Read the model definition and answer for the solid it produces. Units are mm, in the model's axes. Face numbers are marked on the shaded views. Coordinates: 2 decimals unless noted, no trailing zeros. Write each loop counter-clockwise with the first axis right and the second up, starting at its lowest first coordinate (ties: lowest second). Pieces come first, ordered by that corner, then holes.
1) The part is cut by section C-C (z = 1.5). Determine the outline of the cut face in (x, y).
2) Each of these flat-tipped pins is pushed along its axis until it touches: pin 1 Ø5 at (x, y) = (95.5, 15.5) entering from +Z; pin 2 Ø6 at (y, z) = (24.5, 3) entering from +X. Where does it stop, or does it pass through?
3) The part is cut by section A-A (x = 15). Determine the outline of the cut face in (y, z), then the cut area to 3 significant figures.
4) Determine the mould class of the marked faces 1, 2 and 3 for opening direction Z: +Z half, -Z half, draft (parallel to the pull), parting line (faces both ways), or undercut.
5) The part is cut by section D-D (y = 27). Determine the outline of the cut face in (x, z).
6) The part is cut by section B-B (y = 15). Determine the outline of the cut face in (x, z).
7) Find the intervals of material crossed by line 1 (Z direction, x = 46.5, y = 12); line 2 (Y direction, x = 15, z = 1); line 3 (Y direction, x = 9, z = 2.25), in increasing order.
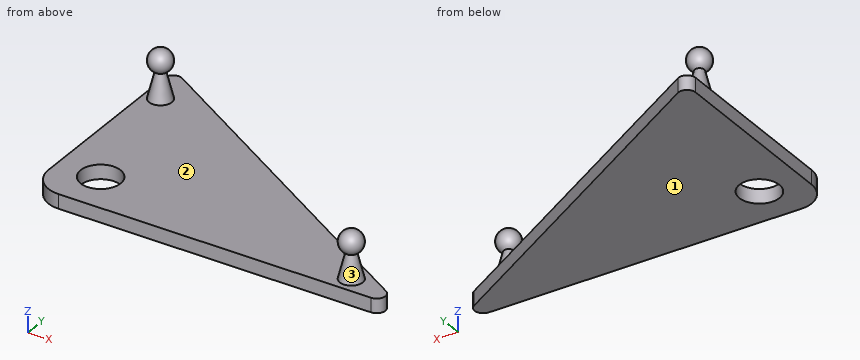
from build123d import *

# Parameters (mm, degrees)
ESTRUSIONE_ESTRUSIONE1_DEPTH = 5
SCHIZZO2_R                   = 7
TAGLIO_ESTRUSIONE1_DEPTH     = 152.6871781
RACCORDO1_R                  = 10
SCHIZZO3_R                   = 4
ESTRUSIONE_ESTRUSIONE2_DEPTH = 10
ESTRUSIONE_ESTRUSIONE2_TAPER = 14
RACCORDO2_R                  = 3
SCHIZZO6_R                   = 4
ESTRUSIONE_ESTRUSIONE3_DEPTH = 10
ESTRUSIONE_ESTRUSIONE3_TAPER = 14


with BuildPart() as part:
    # Schizzo1 → Estrusione-Estrusione1 (new body)
    with BuildSketch(Plane.XY):
        Polygon((0, 0), (0, 78), (130, 0), align=None)
    extrude(amount=ESTRUSIONE_ESTRUSIONE1_DEPTH)

    # Schizzo2 → Taglio-Estrusione1 (cut, through all)
    with BuildSketch(Plane(origin=(0, 0, 0), x_dir=(-1, 0, 0), z_dir=(0, 0, -1))):
        with Locations((-15, 15)):
            Circle(SCHIZZO2_R)
    extrude(amount=-TAGLIO_ESTRUSIONE1_DEPTH, mode=Mode.SUBTRACT)

    # Raccordo1
    raccordo1_edges = [part.edges().sort_by_distance(p)[0] for p in [
        (0, 0, 2.5),
    ]]
    fillet(raccordo1_edges, radius=RACCORDO1_R)

    # Schizzo3 → Estrusione-Estrusione2 (add)
    with BuildSketch(Plane.XY.offset(5)):
        with Locations((5.463985213, 62.137606809)):
            Circle(SCHIZZO3_R)
    extrude(amount=ESTRUSIONE_ESTRUSIONE2_DEPTH, taper=ESTRUSIONE_ESTRUSIONE2_TAPER)

    # Schizzo5 → Rivoluzione1 (revolve)
    with BuildSketch(Plane(origin=(0, 62.137606809, 0), x_dir=(1, 0, 0), z_dir=(0, 1, 0))):
        with BuildLine():
            Line((9.463985213, -18), (1.463985213, -18))
            ThreePointArc((1.463985213, -18), (5.463985213, -22), (9.463985213, -18))
        make_face()
    revolve(axis=Axis((9.463985213, 62.137606809, 18), (-1, 0, 0)))

    # Raccordo2
    raccordo2_edges = [part.edges().sort_by_distance(p)[0] for p in [
        (0, 78, 2.5),
        (130, 0, 2.5),
    ]]
    fillet(raccordo2_edges, radius=RACCORDO2_R)

    # Schizzo6 → Estrusione-Estrusione3 (add)
    with BuildSketch(Plane.XY.offset(5)):
        with Locations((108.33809621, 6)):
            Circle(SCHIZZO6_R)
    extrude(amount=ESTRUSIONE_ESTRUSIONE3_DEPTH, taper=ESTRUSIONE_ESTRUSIONE3_TAPER)

    # Schizzo9 → Rivoluzione3 (revolve)
    with BuildSketch(Plane(origin=(0, 6, 0), x_dir=(1, 0, 0), z_dir=(0, 1, 0))):
        with BuildLine():
            Line((112.33809621, -17.694136404), (104.33809621, -17.694136404))
            ThreePointArc((104.33809621, -17.694136404), (108.33809621, -21.694136404), (112.33809621, -17.694136404))
        make_face()
    revolve(axis=Axis((112.33809621, 6, 17.694136404), (-1, 0, 0)))


solid = part.part
Reported:
1. outline: (0, 10) arc R10 ccw to (10, 0) - (119.17, 0) arc R3 ccw to (120.71, 5.57) - (4.54, 75.27) arc R3 ccw to (0, 72.7) - close; hole circle Ø14 at (15, 15)
2. pin 1: stops at z = 5
2. pin 2: stops at x = 94.17
3. outline: (0, 0) - (8, 0) - (8, 5) - (0, 5) - close; (22, 0) - (69, 0) - (69, 5) - (22, 5) - close
3. area: 275 mm2
4. face 1: -Z half
4. face 2: +Z half
4. face 3: undercut
5. outline: (0, 0) - (85, 0) - (85, 5) - (0, 5) - close
6. outline: (0, 0) - (8, 0) - (8, 5) - (0, 5) - close; (22, 0) - (105, 0) - (105, 5) - (22, 5) - close
7. line 1: z = 0 to 5
7. line 2: y = 0 to 8, 22 to 69
7. line 3: y = 0.05 to 11.39, 18.61 to 72.6
